```python
from build123d import *

# Parameters (mm, degrees)
F1_DEPTH = 1000
F3_DEPTH = 1000
F4_W     = 80
F4_H     = 680.397727
F5_DEPTH = 1000


with BuildPart() as f1:
    # F0 (on Front) → F1 (new body)
    with BuildSketch(Plane.XZ):
        Polygon((0, 800), (0, 0), (660, 0), (660, 975), align=None)
    extrude(amount=F1_DEPTH)

    # F2 (on Front) → F3 (join, through all)
    with BuildSketch(Plane.XZ):
        Polygon((0, 840), (0, 800), (1.5, 800.397727), (1.5, 840), align=None)
    extrude(amount=F3_DEPTH)

    # F4 (on face) → F5 (cut, through all)
    with BuildSketch(Plane(origin=(0, 0, 0), x_dir=(-1, 0, 0), z_dir=(0, 1, 0))):
        with Locations((-40, 340.198863)):
            Rectangle(F4_W, F4_H)
    extrude(amount=-F5_DEPTH, mode=Mode.SUBTRACT)


solid = f1.part
```
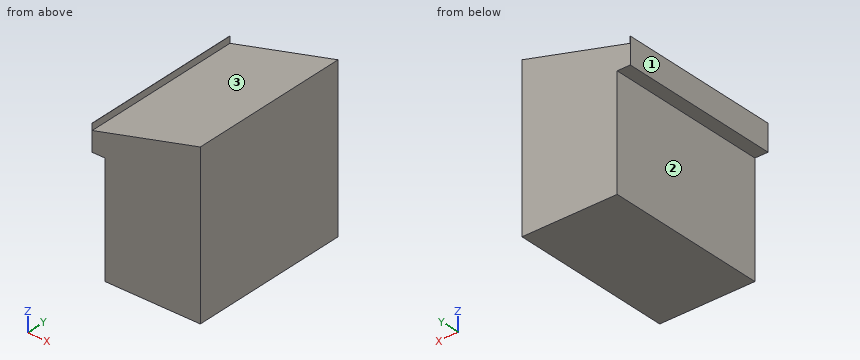
Design review of the part built by this model. Coordinates are the model's own, in mm. Face numbers are marked on the shaded views. A direction names the side the tool comes from. Round coordinates to 2 decimals unless told otherwise and drop trailing zeros. Write each loop counter-clockwise with the first axis right and the second up, starting at its lowest first coordinate (ties: lowest second). Pieces come first, ordered by that corner, then holes.
Item 1: We need section A-A on y = -690. Write out the cut boundary in (x, z).
Item 2: We need section B-B on x = 561. Write out the cut boundary in (y, z).
Item 3: For the marked faces 1, 2 and 3, list the 3-axis set-ups (+Z, -Z, +X, -X, +Y, -Y) from which the entire face can be reached by the end or side of a thin tool; tool diameter is ignored.
Item 4: We need section C-C on z = 425.5. Write out the cut boundary in (x, y).
Item 5: For probe 1 along X at (y, z) = (-497, 284.5); probe 2 along Z at (x, y) = (534, -751.5); probe 3 along Z at (x, y) = (123.5, -344.5), list the stretches that pass through material, from the lowest coordinate up.
Item 6: Clearance check with flat-ended pins moving along their axes: pin 1 Ø3 at (x, y) = (252.5, -748.5) entering from +Z; pin 2 Ø10 at (x, y) = (153.5, -606) entering from +Z; pin 3 Ø1.2 at (x, y) = (1, -733) entering from +Z. State where each tip first meets the part, or that it passes through.
Returned:
1. outline: (0, 680.4) - (80, 680.4) - (80, 0) - (660, 0) - (660, 975) - (1.5, 800.4) - (1.5, 840) - (0, 840) - close
2. outline: (-1000, 0) - (0, 0) - (0, 948.75) - (-1000, 948.75) - close
3. face 1: +Z, -Z, -X, +Y, -Y
3. face 2: -Z, -X, +Y, -Y
3. face 3: +Z, +Y, -Y
4. outline: (80, -1000) - (660, -1000) - (660, 0) - (80, 0) - close
5. probe 1: x = 80 to 660
5. probe 2: z = 0 to 941.59
5. probe 3: z = 0 to 832.75
6. pin 1: stops at z = 867.35
6. pin 2: stops at z = 842.03
6. pin 3: stops at z = 840
